Read the model definition and answer for the solid it produces. Units are mm, in the model's axes. Face numbers are marked on the shaded views. Coordinates: 2 decimals unless noted, no trailing zeros. Order: outer loops, then holes, each group sorted by start corner. A loop starts at its lowest first (then second) coordinate and runs counter-clockwise, first axis right, second up. Notation, with made-up numbers: (36.25, 55) -> (72.25, 55) arc R26 ccw to (72.25, 90) -> close; hole circle Ø10 at (89, 6.5). An arc over 180 degrees is marked (long way). Answer as a JSON object with one key per item and string values. Group by question number.
1) Section A-A on x = 0 is taken. Determine the outline of the cut face in (y, z).
2) Given pin 1 (12 mm diameter, centred on x = 16.5, y = 47, fed in from -Z); pin 2 (1 mm diameter, centred on y = -48, z = -7.5, fed in from -X); pin 3 (4 mm diameter, centred on x = -29, z = -26, fed in from -Y), each flat-ended and moving along its own axis, determine where each tip first touches the part or whether it passes through.
3) Determine the mould class of the marked faces 1, 2 and 3 for opening direction Z: released by +Z, released by -Z, zero draft, split by the parting line, or undercut.
4) Consider L1, parallel to Z at x = -20, y = 16; L2, parallel to Y at x = -16, z = 8; L3, parallel to Y at x = 0, z = 21. Determine where each line is inside the solid, lowest interval first.
5) Section B-B on z = -18.5 is taken. Determine the outline of the cut face in (x, y).
from build123d import *

# Parameters (mm, degrees)
BOSS_EXTRUDE1_DEPTH = 10
CHAMFER2_SIZE       = 5
SKETCH4_R           = 20
SKETCH4_R_2         = 25
BOSS_EXTRUDE2_DEPTH = 30


with BuildPart() as part:
    # Sketch2 → Boss-Extrude1 (new body)
    with BuildSketch(Plane.XY.offset(25)):
        with BuildLine():
            ThreePointArc((20.777841167, 66.366847826), (9.632079925, 95.3340364), (-19.842240524, 85.608274648))
            ThreePointArc((-19.842240524, 85.608274648), (-43.263152194, 0.334990999), (-27.623511317, -86.702205882))
            ThreePointArc((-27.623511317, -86.702205882), (12.846707304, -102.110184644), (26.549463713, -61.03125))
            ThreePointArc((26.549463713, -61.03125), (9.450478546, 2.023887612), (20.777841167, 66.366847826))
        make_face()
    extrude(amount=BOSS_EXTRUDE1_DEPTH)

    # Chamfer2
    chamfer2_edges = [part.edges().sort_by_distance(p)[0] for p in [
        (9.450478546, 2.023887612, 35),
        (9.632079925, 95.3340364, 35),
        (-43.263152194, 0.334990999, 35),
        (12.846707304, -102.110184644, 35),
    ]]
    chamfer(chamfer2_edges, length=CHAMFER2_SIZE)

    # Sketch4 → Boss-Extrude2 (add)
    with BuildSketch(Plane(origin=(0, 0, 25), x_dir=(-1, 0, 0), z_dir=(0, 0, -1))):
        with Locations((0, 75)):
            Circle(SKETCH4_R)
        with Locations((0, -75)):
            Circle(SKETCH4_R_2)
    extrude(amount=BOSS_EXTRUDE2_DEPTH)

    # Mirror3: part across plane


with BuildPart() as part_1:
    add(part.part)
    add(part.part.mirror(Plane.XY))


solid = part_1.part
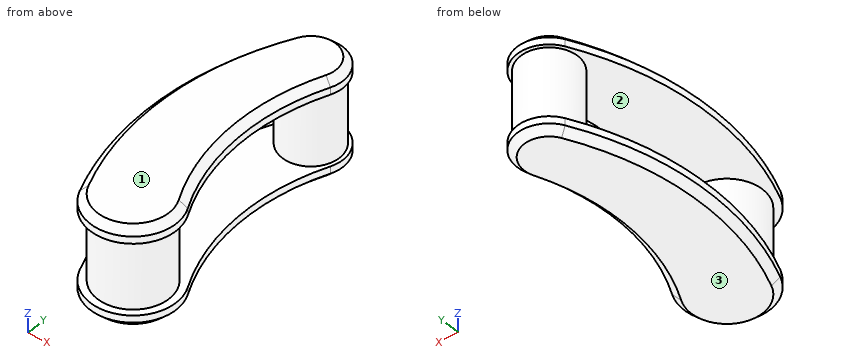
Worked answers:
{
 "1": {"outline": "(-105, -30) -> (-100, -35) -> (92.5, -35) -> (97.5, -30) -> (97.5, -25) -> (95, -25) -> (95, 25) -> (97.5, 25) -> (97.5, 30) -> (92.5, 35) -> (-100, 35) -> (-105, 30) -> (-105, 25) -> (-100, 25) -> (-100, -25) -> (-105, -25) -> close; hole (-50, -25) -> (55, -25) -> (55, 25) -> (-50, 25) -> close"},
 "2": {"pin 1": "stops at z = -33.81", "pin 2": "passes through", "pin 3": "stops at y = -88.08"},
 "3": {"face 1": "released by +Z", "face 2": "undercut", "face 3": "released by -Z"},
 "4": {"L1": "z = -35 to -25, 25 to 35", "L2": "y = -94.21 to -55.79, 63 to 87", "L3": "y = -100 to -50, 55 to 95"},
 "5": {"outline": "circle Ø50 at (0, -75); circle Ø40 at (0, 75)"}
}
